```python
from build123d import *

# Parameters (mm, degrees)
SKETCH1_W            = 64.77
SKETCH1_H            = 48.006
SKETCH1_W_2          = 58.674
SKETCH1_H_2          = 40.386
BOSS_EXTRUDE1_DEPTH  = 12.7
BOSS_EXTRUDE2_DEPTH  = 3.175
BOSS_EXTRUDE3_DEPTH  = 21.7932
SKETCH6_W            = 22.86
SKETCH6_H            = 2.667
SKETCH6_H_2          = 5.08
CUT_EXTRUDE1_DEPTH   = 103.235990753
SKETCH7_W            = 22.86
SKETCH7_H            = 3.81
SKETCH7_H_2          = 1.143
CUT_EXTRUDE2_DEPTH   = 12.7
SKETCH10_W           = 13.97
SKETCH10_H           = 3.81
BOSS_EXTRUDE4_DEPTH  = 5.08
BOSS_EXTRUDE5_DEPTH  = 3.81
SKETCH12_R           = 1.27
CUT_EXTRUDE3_DEPTH   = 110.514697261
BOSS_EXTRUDE7_DEPTH  = 3.81
SKETCH14_W           = 13.97
SKETCH14_H           = 3.81
BOSS_EXTRUDE8_DEPTH  = 5.08
SKETCH15_R           = 1.27
CUT_EXTRUDE4_DEPTH   = 114.762270179
BOSS_EXTRUDE9_DEPTH  = 3.81
BOSS_EXTRUDE10_DEPTH = 3.81
SKETCH21_W           = 58.42
SKETCH21_H           = 5.08
SKETCH21_W_2         = 24.109012503
SKETCH21_H_2         = 2.54
SKETCH21_W_3         = 11.450987497
BOSS_EXTRUDE13_DEPTH = 3.81
BOSS_EXTRUDE14_DEPTH = 24.109012503
BOSS_EXTRUDE15_DEPTH = 11.450987497


with BuildPart() as part:
    # Sketch1 → Boss-Extrude1 (new body)
    with BuildSketch(Plane.XY):
        Rectangle(SKETCH1_W, SKETCH1_H)
        Rectangle(SKETCH1_W_2, SKETCH1_H_2, mode=Mode.SUBTRACT)
    extrude(amount=BOSS_EXTRUDE1_DEPTH)

    # Sketch3 → Boss-Extrude2 (add)
    with BuildSketch(Plane.XY.offset(12.7)):
        Polygon((79.354012503, -24.003), (79.354012503, -20.828), (56.494012503, -20.828), (56.494012503, -24.003), (-32.385, -24.003), (-32.385, 28.067), (56.494012503, 28.067), (56.494012503, 25.527), (79.354012503, 25.527), (79.354012503, 28.067), (90.805, 28.067), (90.805, -24.003), align=None)
    extrude(amount=BOSS_EXTRUDE2_DEPTH)

    # Sketch5 → Boss-Extrude3 (add)
    with BuildSketch(Plane.XY.offset(15.875)):
        Polygon((56.494012503, 28.067), (-32.385, 28.067), (-32.385, -24.003), (56.494012503, -24.003), (56.494012503, -18.923), (-27.305, -18.923), (-27.305, 25.4), (56.494012503, 25.4), align=None)
        Polygon((88.011, -18.923), (79.354012503, -18.923), (79.354012503, -24.003), (90.805, -24.003), (90.805, 19.177), (88.011, 19.177), align=None)
    extrude(amount=BOSS_EXTRUDE3_DEPTH)

    # Sketch6 → Cut-Extrude1 (cut, through all)
    with BuildSketch(Plane.XY.offset(37.6682)):
        with Locations((3.175, 26.7335)):
            Rectangle(SKETCH6_W, SKETCH6_H)
        with Locations((3.175, -21.463)):
            Rectangle(SKETCH6_W, SKETCH6_H_2)
    extrude(amount=-CUT_EXTRUDE1_DEPTH, mode=Mode.SUBTRACT)

    # Sketch7 → Cut-Extrude2 (cut)
    with BuildSketch(Plane(origin=(0, 0, 0), x_dir=(-1, 0, 0), z_dir=(0, 0, -1))):
        with Locations((-3.175, 22.098)):
            Rectangle(SKETCH7_W, SKETCH7_H)
        with Locations((-3.175, -20.7645)):
            Rectangle(SKETCH7_W, SKETCH7_H_2)
    extrude(amount=-CUT_EXTRUDE2_DEPTH, mode=Mode.SUBTRACT)

    # Sketch10 → Boss-Extrude4 (add)
    with BuildSketch(Plane.ZY.offset(32.385)):
        with Locations((30.6832, -22.098)):
            Rectangle(SKETCH10_W, SKETCH10_H)
    extrude(amount=BOSS_EXTRUDE4_DEPTH)

    # Sketch11 → Boss-Extrude5 (add)
    with BuildSketch(Plane.XY.offset(37.6682)):
        Polygon((-37.465, -20.193), (-32.385, -20.193), (-32.385, -15.113), align=None)
    extrude(amount=-BOSS_EXTRUDE5_DEPTH)

    # Sketch12 → Cut-Extrude3 (cut, through all)
    with BuildSketch(Plane(origin=(0, -20.193, 0), x_dir=(1, 0, 0), z_dir=(0, 1, 0))):
        with Locations(Location((-34.925, -30.6832, 0), (0, 0, 270))):
            Circle(SKETCH12_R)
    extrude(amount=-CUT_EXTRUDE3_DEPTH, mode=Mode.SUBTRACT)

    # Sketch13 → Boss-Extrude7 (add)
    with BuildSketch(Plane(origin=(0, 0, 23.6982), x_dir=(-1, 0, 0), z_dir=(0, 0, -1))):
        Polygon((32.385, -15.113), (32.385, -20.193), (37.465, -20.193), align=None)
    extrude(amount=-BOSS_EXTRUDE7_DEPTH)

    # Sketch14 → Boss-Extrude8 (add)
    with BuildSketch(Plane(origin=(90.805, 0, 0), x_dir=(0, 0, -1), z_dir=(1, 0, 0))):
        with Locations((-30.6832, -22.098)):
            Rectangle(SKETCH14_W, SKETCH14_H)
    extrude(amount=BOSS_EXTRUDE8_DEPTH)

    # Sketch15 → Cut-Extrude4 (cut, through all)
    with BuildSketch(Plane(origin=(0, -20.193, 0), x_dir=(1, 0, 0), z_dir=(0, 1, 0))):
        with Locations(Location((93.345, -30.6832, 0), (0, 0, 270))):
            Circle(SKETCH15_R)
    extrude(amount=-CUT_EXTRUDE4_DEPTH, mode=Mode.SUBTRACT)

    # Sketch17 → Boss-Extrude9 (add)
    with BuildSketch(Plane.XY.offset(37.6682)):
        Polygon((95.885, -20.193), (90.805, -20.193), (90.805, -15.113), align=None)
    extrude(amount=-BOSS_EXTRUDE9_DEPTH)

    # Sketch18 → Boss-Extrude10 (add)
    with BuildSketch(Plane(origin=(0, 0, 23.6982), x_dir=(-1, 0, 0), z_dir=(0, 0, -1))):
        Polygon((-95.885, -20.193), (-90.805, -20.193), (-90.805, -15.113), align=None)
    extrude(amount=-BOSS_EXTRUDE10_DEPTH)

    # Sketch21 → Boss-Extrude13 (add)
    with BuildSketch(Plane(origin=(0, 0, 12.7), x_dir=(-1, 0, 0), z_dir=(0, 0, -1))):
        with Locations((-61.595, 12.5095)):
            Rectangle(SKETCH21_W, SKETCH21_H)
        with Locations((-61.595, -8.4455)):
            Rectangle(SKETCH21_W, SKETCH21_H)
        with Locations((-44.439506252, -22.733)):
            Rectangle(SKETCH21_W_2, SKETCH21_H_2)
        with Locations((-85.079506252, -22.733)):
            Rectangle(SKETCH21_W_3, SKETCH21_H_2)
    extrude(amount=BOSS_EXTRUDE13_DEPTH)

    # Sketch22 → Boss-Extrude14 (add)
    with BuildSketch(Plane(origin=(56.494012503, 0, 0), x_dir=(0, 0, -1), z_dir=(1, 0, 0))):
        Polygon((-8.89, -21.463), (-12.7, -21.463), (-12.7, -18.923), align=None)
    extrude(amount=-BOSS_EXTRUDE14_DEPTH)

    # Sketch23 → Boss-Extrude15 (add)
    with BuildSketch(Plane(origin=(90.805, 0, 0), x_dir=(0, 0, -1), z_dir=(1, 0, 0))):
        Polygon((-8.89, -21.463), (-12.7, -21.463), (-12.7, -18.923), align=None)
    extrude(amount=-BOSS_EXTRUDE15_DEPTH)


solid = part.part
```
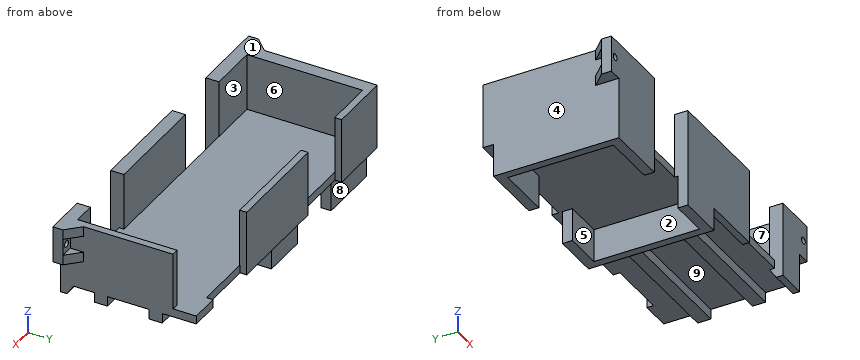
Input: part model. Units: mm. Frame: model coordinates. Face numbers are marked on the shaded views. A direction names the side the tool comes from. Round coordinates to 2 decimals unless told otherwise and drop trailing zeros. Loops run counter-clockwise (first coordinate to the right, second up) from the corner with the lowest first, then second, coordinate; pieces in that order, holes last. Notation, with made-up numbers: (7.5, -14) -> (39.5, -14) arc R18 cw to (39.5, 8) -> close; hole circle Ø9 at (77, 3). An arc over 180 degrees is marked (long way). Use one line per item in the form item = value. Start each with the question number.
Item 1: Contact query for flat-ended pins moving along their axis: pin 1 Ø5.5 at (x, y) = (70.5, -7.5) entering from -Z; pin 2 Ø12 at (x, y) = (79, 3) entering from +Z (3 decimals); pin 3 Ø4 at (x, z) = (70.5, 10.5) entering from -Y; pin 4 Ø5 at (x, z) = (-3.5, 7.5) entering from +Y. Output: stop coordinate, or through.
Item 2: Mould query, pull axis X, two halves, no side actions, for the marked faces 1, 2, 3 and 4. Classes: pulls with the +X half, pulls with the -X half, needs draft (parallel to the pull), parting line crosses it, or undercut.
Item 3: Section query D-D on y = 3. Return the cut outline in (x, z) (3 decimals), then the cut area to 3 significant figures.
Item 4: Set-up query: the marked faces 5, 6, 7, 8 and 9. Return all of +Z, -Z, +X, -X, +Y, -Y with unobstructed straight access to the full face (end or side cutting, diameter ignored); none if empty.
Item 5: Material intervals for L1, parallel to X at y = 18, z = 9 (3 decimals); L2, parallel to Y at x = -20, z = 27.5; L3, parallel to X at y = 9.5, z = 23.5 (3 decimals), sorted ascending. Write a range as from..to.
Item 6: Section query A-A on z = 17.5. Return the cut outline in (x, y) (3 decimals), then the cut area to 3 significant figures.
Item 7: Section query B-B on z = 7.5. Return the cut outline in (x, y) (3 decimals).
Item 8: Section query C-C on x = 76.5. Return the cut outline in (y, z) (1 decimal), then the cut area to 3 significant figures.
Ans:
q1.pin_1 = 8.89
q1.pin_2 = 15.875
q1.pin_3 = -10.99
q1.pin_4 = through
q2.face_1 = needs draft
q2.face_2 = undercut
q2.face_3 = undercut
q2.face_4 = pulls with the -X half
q3.outline = (-32.385, 0) -> (-29.337, 0) -> (-29.337, 12.7) -> (29.337, 12.7) -> (29.337, 0) -> (32.385, 0) -> (32.385, 12.7) -> (90.805, 12.7) -> (90.805, 37.668) -> (88.011, 37.668) -> (88.011, 15.875) -> (-27.305, 15.875) -> (-27.305, 37.668) -> (-32.385, 37.668) -> close
q3.area = 640 mm^2
q4.face_5 = -Z
q4.face_6 = +Z
q4.face_7 = +Z, +Y
q4.face_8 = -Z, +X, -X, +Y
q4.face_9 = -Z, +X
q5.L1 = -32.385..-29.337, 29.337..32.385
q5.L2 = -24..-18.92, 25.4..28.07
q5.L3 = -32.385..-27.305, 88.011..90.805
q6.outline = (-32.385, -24.003) -> (-8.255, -24.003) -> (-8.255, -18.923) -> (-27.305, -18.923) -> (-27.305, 25.4) -> (-8.255, 25.4) -> (-8.255, 28.067) -> (-32.385, 28.067) -> close; (14.605, -24.003) -> (56.494, -24.003) -> (56.494, -18.923) -> (14.605, -18.923) -> close; (14.605, 25.4) -> (56.494, 25.4) -> (56.494, 28.067) -> (14.605, 28.067) -> close; (79.354, -24.003) -> (90.805, -24.003) -> (90.805, 19.177) -> (88.011, 19.177) -> (88.011, -18.923) -> (79.354, -18.923) -> close
q6.area = 901 mm^2
q7.outline = (-32.385, -24.003) -> (-8.255, -24.003) -> (-8.255, -20.193) -> (-29.337, -20.193) -> (-29.337, 20.193) -> (-8.255, 20.193) -> (-8.255, 24.003) -> (-32.385, 24.003) -> close; (14.605, -24.003) -> (32.385, -24.003) -> (32.385, 24.003) -> (14.605, 24.003) -> (14.605, 20.193) -> (29.337, 20.193) -> (29.337, -20.193) -> (14.605, -20.193) -> close
q8.outline = (-20.8, 12.7) -> (-11, 12.7) -> (-11, 8.9) -> (-5.9, 8.9) -> (-5.9, 12.7) -> (10, 12.7) -> (10, 8.9) -> (15, 8.9) -> (15, 12.7) -> (25.5, 12.7) -> (25.5, 15.9) -> (-20.8, 15.9) -> close
q8.area = 186 mm^2
